from build123d import *

# Parameters (mm, degrees)
SKETCH3_R           = 29.0195
SKETCH3_R_2         = 24.765
BOSS_EXTRUDE2_DEPTH = 2.54
SKETCH4_R           = 32.8295
SKETCH4_R_2         = 29.0195
BOSS_EXTRUDE3_DEPTH = 9.5504
BOSS_EXTRUDE4_START = 18.415
SKETCH5_R           = 32.8295
SKETCH5_R_2         = 27.5082
BOSS_EXTRUDE4_DEPTH = 18.415


with BuildPart() as part:
    # Sketch3 → Boss-Extrude2 (new body)
    with BuildSketch(Plane(origin=(0, 0, 0), x_dir=(1, 0, 0), z_dir=(0, 1, 0))):
        with Locations(Location((0, 0, 0), (0, 0, 270))):
            Circle(SKETCH3_R)
        with Locations(Location((0, 0, 0), (0, 0, 270))):
            Circle(SKETCH3_R_2, mode=Mode.SUBTRACT)
    extrude(amount=BOSS_EXTRUDE2_DEPTH)

    # Sketch4 → Boss-Extrude3 (add)
    with BuildSketch(Plane(origin=(0, 0, 0), x_dir=(1, 0, 0), z_dir=(0, 1, 0))):
        with Locations(Location((0, 0, 0), (0, 0, 90))):
            Circle(SKETCH4_R)
        with Locations(Location((0, 0, 0), (0, 0, 90))):
            Circle(SKETCH4_R_2, mode=Mode.SUBTRACT)
    extrude(amount=BOSS_EXTRUDE3_DEPTH)

    # Sketch5 → Boss-Extrude4 (add)
    with BuildSketch(Plane.XZ.offset(BOSS_EXTRUDE4_START)):
        with Locations(Location((0, 0, 0), (0, 0, 270))):
            Circle(SKETCH5_R)
        with Locations(Location((0, 0, 0), (0, 0, 270))):
            Circle(SKETCH5_R_2, mode=Mode.SUBTRACT)
    extrude(amount=-BOSS_EXTRUDE4_DEPTH)


solid = part.part
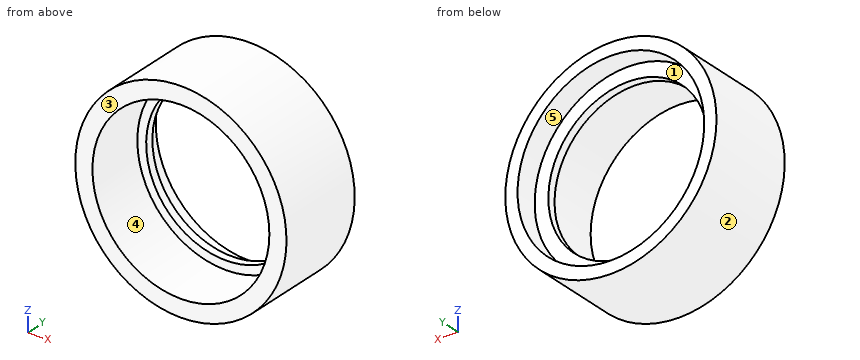
The listing builds one solid part. Answer for the finished solid, in the listing's coordinates (mm). Face numbers are marked on the shaded views. A direction names the side the tool comes from. Coordinates: 2 decimals unless noted, no trailing zeros. Write each loop counter-clockwise with the first axis right and the second up, starting at its lowest first coordinate (ties: lowest second). Pieces come first, ordered by that corner, then holes. Notation, with made-up numbers: M 16,84.5 L 33,84.5 A16 cw 33,99.5 Z; hole C 45.5,12.5 d10. An arc over 180 degrees is marked long. Write each question's results on one line, items separated by ' | '.
Item 1: For a pull along X with two mould halves and no side action, classify the marked faces 1, 2 and 3 as released by +X, released by -X, zero draft, split by the parting line, or undercut.
Answer below:
face 1: undercut | face 2: split by the parting line | face 3: zero draft
Item 2: Which of the six approach directions +Z, -Z, +X, -X, +Y, -Y give full straight-line access (tool end or side, diameter ignored) to the marked faces 4 and 5?
Answer below:
face 4: -Y | face 5: +Y
Item 3: The part is cut by section C-C on y = -2. Determine the outline of the cut face in (x, z), and give its area (3 significant figures).
Answer below:
outline: C 0,0 d65.66; hole C 0,0 d55.02 | area: 1,010 mm2
Item 4: The part is cut by section A-A on z = 0. Determine the outline of the cut face in (x, y) (1 decimal), and give its area (3 significant figures).
Answer below:
outline: M -32.8,-18.4 L -27.5,-18.4 L -27.5,0 L -24.8,0 L -24.8,2.5 L -29,2.5 L -29,9.6 L -32.8,9.6 Z; M 24.8,0 L 27.5,0 L 27.5,-18.4 L 32.8,-18.4 L 32.8,9.6 L 29,9.6 L 29,2.5 L 24.8,2.5 Z | area: 290 mm2
Item 5: Given P1, Ø1, axis at y = -9.5, z = -25.5, coming from the +X side; P2, Ø6, axis at x = -3.5, y = -14, coming from the -Z side; P3, Ø3, axis at y = 4, z = 23.5, coming from the +X side; P4, Ø5, axis at x = 18, z = -10.5, coming from the +Y side, each flat-ended and moving along its own axis, determine where each tip first touches the part or whether it passes through.
Answer below:
P1: x = 21.28 | P2: z = -32.83 | P3: x = 24.37 | P4: through
Item 6: The part is cut by section B-B on x = 0. Determine the outline of the cut face in (y, z) (1 decimal).
Answer below:
outline: M -18.4,-32.8 L 9.6,-32.8 L 9.6,-29 L 2.5,-29 L 2.5,-24.8 L 0,-24.8 L 0,-27.5 L -18.4,-27.5 Z; M -18.4,27.5 L 0,27.5 L 0,24.8 L 2.5,24.8 L 2.5,29 L 9.6,29 L 9.6,32.8 L -18.4,32.8 Z
Item 7: Consider probe 1 along X at (y, z) = (5.75, 0); probe 2 along Y at (x, z) = (23.5, 15.5) (3 decimals). Determine where each line is inside the solid, lowest interval first. Write a range as [from, to].
Answer below:
probe 1: [-32.83, -29.02], [29.02, 32.83] | probe 2: [-18.415, 2.54]
